CAD build for the part. Positions are in the model's coordinates, mm. Round coordinates to 2 decimals unless told otherwise and drop trailing zeros. Loops run counter-clockwise (first coordinate to the right, second up) from the corner with the lowest first, then second, coordinate; pieces in that order, holes last. Notation, with made-up numbers: M 15,56 L 39,56 A31 ccw 39,83 Z; hole C 71,2.25 d3. An arc over 180 degrees is marked long. Use a Markdown table: item, result. Add a question column.
(1) Flat gauge pin, fed straight in: P1, Ø2.5, axis at x = 52.41, y = -5.46, coming from the -Z side. Where does the tip first touch, or does it go through?
(2) Wall check: L1, parallel to Y at x = 75, z = 5.75; L2, parallel to Y at x = -65, z = 3.75; L3, parallel to X at y = -50, z = 4.25. Give the ranges that are in metal, low to high.
(3) Band-saw the part on A-A, the plane x = 75. Write the cut outline in (y, z), and give its area (3 significant figures).
from build123d import *

# Parameters (mm, degrees)
F0_W     = 160
F0_H     = 130
F0_R     = 2
F0_R_2   = 1.8
F0_R_3   = 1.25
F0_R_4   = 0.85
F1_DEPTH = 10


with BuildPart() as f1:
    # F0 (on Top) → F1 (new body)
    with BuildSketch(Plane.XY):
        Rectangle(F0_W, F0_H)
        with Locations((-75, -53)):
            Circle(F0_R, mode=Mode.SUBTRACT)
        with Locations((-64.008, -55.753)):
            Circle(F0_R_2, mode=Mode.SUBTRACT)
        with Locations((-64.008, -49.753)):
            Circle(F0_R_3, mode=Mode.SUBTRACT)
        with Locations((-57.062, -57.54)):
            Circle(F0_R_4, mode=Mode.SUBTRACT)
        with Locations((-51.562, -57.54)):
            Circle(F0_R_4, mode=Mode.SUBTRACT)
        with Locations((-45.719, -29.21)):
            Circle(F0_R_4, mode=Mode.SUBTRACT)
        with Locations((62.484, -54.229)):
            Circle(F0_R_2, mode=Mode.SUBTRACT)
        with Locations((75, -53)):
            Circle(F0_R, mode=Mode.SUBTRACT)
        with Locations((52.412, -34.86099)):
            Circle(F0_R_4, mode=Mode.SUBTRACT)
        with Locations((57.912, -34.86099)):
            Circle(F0_R_4, mode=Mode.SUBTRACT)
        with Locations((62.484, -48.229)):
            Circle(F0_R_3, mode=Mode.SUBTRACT)
        with Locations((52.412, -30.66099)):
            Circle(F0_R_4, mode=Mode.SUBTRACT)
        with Locations((57.912, -30.66099)):
            Circle(F0_R_4, mode=Mode.SUBTRACT)
        with Locations((52.412, -26.46099)):
            Circle(F0_R_4, mode=Mode.SUBTRACT)
        with Locations((57.912, -26.46099)):
            Circle(F0_R_4, mode=Mode.SUBTRACT)
        with Locations((52.412, -22.26099)):
            Circle(F0_R_4, mode=Mode.SUBTRACT)
        with Locations((57.912, -22.26099)):
            Circle(F0_R_4, mode=Mode.SUBTRACT)
        with Locations((52.412, -18.06099)):
            Circle(F0_R_4, mode=Mode.SUBTRACT)
        with Locations((57.912, -18.06099)):
            Circle(F0_R_4, mode=Mode.SUBTRACT)
        with Locations((52.412, -13.86099)):
            Circle(F0_R_4, mode=Mode.SUBTRACT)
        with Locations((57.912, -13.86099)):
            Circle(F0_R_4, mode=Mode.SUBTRACT)
        with Locations((52.412, -9.66099)):
            Circle(F0_R_4, mode=Mode.SUBTRACT)
        with Locations((57.912, -9.66099)):
            Circle(F0_R_4, mode=Mode.SUBTRACT)
        with Locations((52.412, -5.46099)):
            Circle(F0_R_4, mode=Mode.SUBTRACT)
        with Locations((57.912, -5.46099)):
            Circle(F0_R_4, mode=Mode.SUBTRACT)
        with Locations((-63.246, 44.323)):
            Circle(F0_R_4, mode=Mode.SUBTRACT)
        with Locations((-75, 53)):
            Circle(F0_R, mode=Mode.SUBTRACT)
        with Locations((-64.008, 50.007)):
            Circle(F0_R_3, mode=Mode.SUBTRACT)
        with Locations((-64.008, 56.007)):
            Circle(F0_R_2, mode=Mode.SUBTRACT)
        with Locations((52.412, 0.472)):
            Circle(F0_R_4, mode=Mode.SUBTRACT)
        with Locations((57.912, 0.472)):
            Circle(F0_R_4, mode=Mode.SUBTRACT)
        with Locations((52.412, 4.672)):
            Circle(F0_R_4, mode=Mode.SUBTRACT)
        with Locations((57.912, 4.672)):
            Circle(F0_R_4, mode=Mode.SUBTRACT)
        with Locations((52.412, 8.872)):
            Circle(F0_R_4, mode=Mode.SUBTRACT)
        with Locations((57.912, 8.872)):
            Circle(F0_R_4, mode=Mode.SUBTRACT)
        with Locations((52.412, 13.072)):
            Circle(F0_R_4, mode=Mode.SUBTRACT)
        with Locations((57.912, 13.072)):
            Circle(F0_R_4, mode=Mode.SUBTRACT)
        with Locations((52.412, 17.272)):
            Circle(F0_R_4, mode=Mode.SUBTRACT)
        with Locations((57.912, 17.272)):
            Circle(F0_R_4, mode=Mode.SUBTRACT)
        with Locations((36.957, 43.307)):
            Circle(F0_R_4, mode=Mode.SUBTRACT)
        with Locations((62.484, 47.467)):
            Circle(F0_R_3, mode=Mode.SUBTRACT)
        with Locations((62.484, 53.467)):
            Circle(F0_R_2, mode=Mode.SUBTRACT)
        with Locations((75, 53)):
            Circle(F0_R, mode=Mode.SUBTRACT)
    extrude(amount=F1_DEPTH)


solid = f1.part
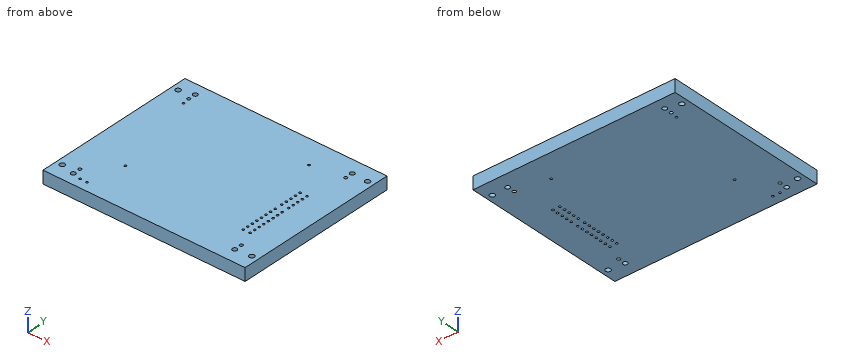
Return value:
| question | item | result |
|---|---|---|
| 1 | P1 | z = 0 |
| 2 | L1 | -65 to -55, -51 to 51, 55 to 65 |
| 2 | L2 | -65 to -57.25, -54.25 to -50.51, -48.99 to 49.25, 50.77 to 54.51, 57.51 to 65 |
| 2 | L3 | -80 to -65.23, -62.78 to 80 |
| 3 | outline | M -65,0 L -55,0 L -55,10 L -65,10 Z; M -51,0 L 51,0 L 51,10 L -51,10 Z; M 55,0 L 65,0 L 65,10 L 55,10 Z |
| 3 | area | 1,220 mm^2 |
